Here's how the part is built. I have some questions about the finished solid (model axes, mm). A direction names the side the tool comes from. Round coordinates to 2 decimals unless told otherwise and drop trailing zeros. Write each loop counter-clockwise with the first axis right and the second up, starting at its lowest first coordinate (ties: lowest second). Pieces come first, ordered by that corner, then holes. Notation, with made-up numbers: (47, 56) - (58, 56) arc R16 cw to (58, 72) - close; hole circle Ø5 at (22.5, 3). An arc over 180 degrees is marked (long way). Write item = value, one per line. Start each with the question number.
Item 1: Which directions (+Z, -Z, +X, -X, +Y, -Y) give clear straight access to the entire face, cutting with the end or side of a thin tool? Please do faces 1 (the face through (-1.5, 0.07, 1.98)), 2 (the face through (0, 1.7, 0)).
Item 2: If we section it at A-A (z = 2.5): Please give me the cut outline in (x, y), and give its area (3 significant figures).
Item 3: For P1, Ø1.5, axis at x = 1, y = 0.5, coming from the +Z side; P2, Ø1.5, axis at y = 0.5, z = 3, coming from the +X side; P3, Ø0.6, axis at y = 1, z = -1, coming from the +X side, each with a flat end and sliding along its axis, tell me the tip position at first contact or that it passes through.
Item 4: If I drill on line 1 along Z through (x, y) = (1.3, 0.8); line 2 along Z through (x, y) = (0.1, -0.1); line 3 along X through (y, z) = (-1.35, 2), over which ranges is the centre line in solid material (lowest first)? Write a range as [from, to].
```python
from build123d import *

# Parameters (mm, degrees)
SKETCH1_R      = 1.75
EXTRUDE1_DEPTH = 0.5
SKETCH2_R      = 1.5
EXTRUDE2_DEPTH = 4
FILLET2_R      = 1
SKETCH4_W      = 13.081078865
SKETCH4_H      = 5.810496129
EXTRUDE3_DEPTH = 1.3
SKETCH5_W      = 0.5
SKETCH5_H      = 0.5
EXTRUDE4_DEPTH = 1.5


with BuildPart() as part:
    # Sketch1 → Extrude1 (new, symmetric)
    with BuildSketch(Plane.XY):
        Circle(SKETCH1_R)
    extrude(amount=EXTRUDE1_DEPTH, both=True)

    # Sketch2 → Extrude2 (add)
    with BuildSketch(Plane.XY.offset(0.5)):
        Circle(SKETCH2_R)
    extrude(amount=EXTRUDE2_DEPTH)

    # Fillet2
    fillet2_edges = [part.edges().sort_by_distance(p)[0] for p in [
        (-1.5, 0, 4.5),
    ]]
    fillet(fillet2_edges, radius=FILLET2_R)

    # Sketch4 → Extrude3 (cut)
    with BuildSketch(Plane(origin=(0, 3, 0), x_dir=(-1, 0, 0), z_dir=(0, 1, 0))):
        with Locations((-1.941605697, 0.17278636)):
            Rectangle(SKETCH4_W, SKETCH4_H)
    extrude3 = extrude(amount=-EXTRUDE3_DEPTH, mode=Mode.SUBTRACT)

    # Sketch5 → Extrude4 (add)
    with BuildSketch(Plane(origin=(0, 0, -0.5), x_dir=(-1, 0, 0), z_dir=(0, 0, -1))):
        with Locations((0, 0.95)):
            Rectangle(SKETCH5_W, SKETCH5_H)
        with Locations((0, -1.05)):
            Rectangle(SKETCH5_W, SKETCH5_H)
    extrude(amount=EXTRUDE4_DEPTH)

    # Simetría1: Extrude3 across plane
    add(extrude3.mirror(Plane.ZX), mode=Mode.SUBTRACT)


solid = part.part
```
Reply:
q1.face_1 = +Z
q1.face_2 = +Z, -Z, +X, -X, +Y
q2.outline = circle Ø3 at (0, 0)
q2.area = 7.07 mm2
q3.P1 = 4.5
q3.P2 = 1.5
q3.P3 = 0.25
q4.line_1 = [-0.5, 0.5]
q4.line_2 = [-0.5, 4.5]
q4.line_3 = [-0.65, 0.65]
